from build123d import *

# Parameters (mm, degrees)
SKETCH_1_W           = 80
SKETCH_1_H           = 75
EXTRUDE_1_DEPTH      = 15
EXTRUDE_2_REACH      = 175.759
EXTRUDE_2_END_RADIUS = 39
SKETCH_2_W           = 45
SKETCH_2_H           = 30
SKETCH_3_R           = 19
EXTRUDE_3_DEPTH      = 62
SKETCH_4_R           = 17.5
CUT_EXTRUDE_1_DEPTH  = 62
SKETCH_6_R           = 5
EXTRUDE_4_DEPTH      = 30
FILLET_1_R           = 3
SKETCH_7_R           = 1.6
CUT_EXTRUDE_3_DEPTH  = 62
SKETCH_5_W           = 78.155385632
SKETCH_5_H           = 2
CUT_EXTRUDE_4_DEPTH  = 62
SKETCH_8_R           = 11
CUT_EXTRUDE_5_DEPTH  = 62
SKETCH_9_R           = 2.5
CUT_EXTRUDE_6_DEPTH  = 118.917343932
SKETCH_10_R          = 2
CUT_EXTRUDE_7_DEPTH  = 118.917343932
SKETCH_11_R          = 2
SKETCH_11_R_2        = 2.5
SKETCH_11_R_3        = 11
CUT_EXTRUDE_8_DEPTH  = 28
SKETCH_12_W          = 72
SKETCH_12_H          = 29.5
EXTRUDE_6_DEPTH      = 2
SKETCH_13_R          = 1.5
CUT_EXTRUDE_9_DEPTH  = 2
SKETCH_14_R          = 1.55
CUT_EXTRUDE_10_DEPTH = 250


with BuildPart() as part:
    # 草图1 → 凸台-拉伸1 (new, symmetric)
    with BuildSketch(Plane(origin=(0, 0, 0), x_dir=(1, 0, 0), z_dir=(0, 1, 0))):
        with BuildLine():
            Line((-40, -37.5), (-40, 37.5))
            ThreePointArc((-40, 37.5), (-68.287857357, 0), (-40, -37.5))
        make_face()
        Rectangle(SKETCH_1_W, SKETCH_1_H)
        with BuildLine():
            Line((40, -37.5), (40, 37.5))
            ThreePointArc((40, 37.5), (62.5, 0), (40, -37.5))
        make_face()
    extrude(amount=EXTRUDE_1_DEPTH, both=True)

    # 凸台-拉伸2: up to this cylinder (the profile starts outside it)
    extrude_2_end = Plane(origin=(-29.287857357, 0, 0), z_dir=(0, -1, 0)) * Cylinder(EXTRUDE_2_END_RADIUS, 430.518, mode=Mode.PRIVATE)
    # 草图2 → 凸台-拉伸2 (add, up to the surface)
    with BuildSketch(Plane(origin=(-106.5, 0, 0), x_dir=(0, 0, -1), z_dir=(1, 0, 0)), mode=Mode.PRIVATE) as extrude_2_sk1:
        Rectangle(SKETCH_2_W, SKETCH_2_H)
    extrude_2_tool1 = extrude(extrude_2_sk1.sketch, amount=EXTRUDE_2_REACH, mode=Mode.PRIVATE) - extrude_2_end
    add(extrude_2_tool1.solids().sort_by_distance((-106.5, 0, 0))[0])

    # 草图3 → 凸台-拉伸3 (add)
    with BuildSketch(Plane.ZY.offset(106.5)):
        Circle(SKETCH_3_R)
    extrude(amount=-EXTRUDE_3_DEPTH)

    # 草图4 → 切除-拉伸1 (cut)
    with BuildSketch(Plane.ZY.offset(106.5)):
        Circle(SKETCH_4_R)
    extrude(amount=-CUT_EXTRUDE_1_DEPTH, mode=Mode.SUBTRACT)

    # 草图6 → 凸台-拉伸4 (add)
    with BuildSketch(Plane(origin=(0, 15, 0), x_dir=(1, 0, 0), z_dir=(0, 1, 0))):
        with Locations((-96.5, 26.5)):
            Circle(SKETCH_6_R)
        with Locations((-76.5, 26.5)):
            Circle(SKETCH_6_R)
    extrude_4 = extrude(amount=-EXTRUDE_4_DEPTH)

    # 圆角1
    fillet_1_edges = [part.edges().sort_by_distance(p)[0] for p in [
        (-99.5, 0, -22.5),
        (-93.5, 0, -22.5),
        (-73.5, 0, -22.5),
        (-79.5, 0, -22.5),
    ]]
    fillet(fillet_1_edges, radius=FILLET_1_R)

    # 镜向3: 凸台-拉伸4 across plane
    add(extrude_4.mirror(Plane.XY))

    # 草图7 → 切除-拉伸3 (cut)
    with BuildSketch(Plane(origin=(0, 15, 0), x_dir=(1, 0, 0), z_dir=(0, 1, 0))):
        with Locations(Location((-96.5, 26.5, 0), (0, 0, 270))):
            Circle(SKETCH_7_R)
        with Locations(Location((-76.5, 26.5, 0), (0, 0, 270))):
            Circle(SKETCH_7_R)
        with Locations(Location((-76.5, -26.5, 0), (0, 0, 270))):
            Circle(SKETCH_7_R)
        with Locations(Location((-96.5, -26.5, 0), (0, 0, 270))):
            Circle(SKETCH_7_R)
    extrude(amount=-CUT_EXTRUDE_3_DEPTH, mode=Mode.SUBTRACT)

    # 草图5 → 切除-拉伸4 (cut)
    with BuildSketch(Plane.ZY.offset(106.5)):
        Rectangle(SKETCH_5_W, SKETCH_5_H)
    extrude(amount=-CUT_EXTRUDE_4_DEPTH, mode=Mode.SUBTRACT)

    # 草图8 → 切除-拉伸5 (cut)
    with BuildSketch(Plane.XZ.offset(15)):
        with Locations(Location((0, 0, 0), (0, 0, 270))):
            Circle(SKETCH_8_R)
    extrude(amount=-CUT_EXTRUDE_5_DEPTH, mode=Mode.SUBTRACT)

    # 草图9 → 切除-拉伸6 (cut, through all)
    with BuildSketch(Plane.XZ.offset(15)):
        with Locations(Location((14, 14, 0), (0, 0, 270))):
            Circle(SKETCH_9_R)
        with Locations(Location((14, -14, 0), (0, 0, 270))):
            Circle(SKETCH_9_R)
        with Locations(Location((-14, -14, 0), (0, 0, 270))):
            Circle(SKETCH_9_R)
        with Locations(Location((-14, 14, 0), (0, 0, 270))):
            Circle(SKETCH_9_R)
    extrude(amount=-CUT_EXTRUDE_6_DEPTH, mode=Mode.SUBTRACT)

    # 草图10 → 切除-拉伸7 (cut, through all)
    with BuildSketch(Plane(origin=(0, 15, 0), x_dir=(1, 0, 0), z_dir=(0, 1, 0))):
        with Locations(Location((32.5, 32.5, 0), (0, 0, 270))):
            Circle(SKETCH_10_R)
        with Locations(Location((-32.5, 32.5, 0), (0, 0, 270))):
            Circle(SKETCH_10_R)
        with Locations(Location((-32.5, -32.5, 0), (0, 0, 270))):
            Circle(SKETCH_10_R)
        with Locations(Location((32.5, -32.5, 0), (0, 0, 270))):
            Circle(SKETCH_10_R)
    extrude(amount=-CUT_EXTRUDE_7_DEPTH, mode=Mode.SUBTRACT)

    # 草图11 → 切除-拉伸8 (cut)
    with BuildSketch(Plane.XZ.offset(15)):
        with BuildLine():
            Line((-44.5, 9.013878189), (-44.5, 0))
            Line((-44.5, 0), (-44.5, -9.013878189))
            Line((-44.5, -9.013878189), (-44.5, -11.66190379))
            Line((-44.5, -11.66190379), (-44.5, -33.728188748))
            ThreePointArc((-44.5, -33.728188748), (-42.138664615, -34.696638927), (-39.716184164, -35.5))
            Line((-39.716184164, -35.5), (39.49358869, -35.5))
            ThreePointArc((39.49358869, -35.5), (60.5, 0), (39.49358869, 35.5))
            Line((39.49358869, 35.5), (-39.716184164, 35.5))
            ThreePointArc((-39.716184164, 35.5), (-42.138664615, 34.696638927), (-44.5, 33.728188748))
            Line((-44.5, 33.728188748), (-44.5, 11.66190379))
            Line((-44.5, 11.66190379), (-44.5, 9.013878189))
        make_face()
        with Locations(Location((-32.5, -32.5, 0), (0, 0, 90))):
            Circle(SKETCH_11_R, mode=Mode.SUBTRACT)
        with Locations(Location((-14, -14, 0), (0, 0, 270))):
            Circle(SKETCH_11_R_2, mode=Mode.SUBTRACT)
        with Locations(Location((32.5, -32.5, 0), (0, 0, 90))):
            Circle(SKETCH_11_R, mode=Mode.SUBTRACT)
        with Locations(Location((14, -14, 0), (0, 0, 270))):
            Circle(SKETCH_11_R_2, mode=Mode.SUBTRACT)
        with Locations(Location((0, 0, 0), (0, 0, 270))):
            Circle(SKETCH_11_R_3, mode=Mode.SUBTRACT)
        with Locations(Location((-14, 14, 0), (0, 0, 270))):
            Circle(SKETCH_11_R_2, mode=Mode.SUBTRACT)
        with Locations(Location((-32.5, 32.5, 0), (0, 0, 90))):
            Circle(SKETCH_11_R, mode=Mode.SUBTRACT)
        with Locations(Location((14, 14, 0), (0, 0, 270))):
            Circle(SKETCH_11_R_2, mode=Mode.SUBTRACT)
        with Locations(Location((32.5, 32.5, 0), (0, 0, 90))):
            Circle(SKETCH_11_R, mode=Mode.SUBTRACT)
    extrude(amount=-CUT_EXTRUDE_8_DEPTH, mode=Mode.SUBTRACT)

    # 草图12 → 凸台-拉伸6 (add)
    with BuildSketch(Plane.XZ.offset(15)):
        with BuildLine():
            Line((-44.5, 11.66190379), (-44.5, -11.66190379))
            Line((-44.5, -11.66190379), (-44.5, -33.728188748))
            ThreePointArc((-44.5, -33.728188748), (-42.138664615, -34.696638927), (-39.716184164, -35.5))
            Line((-39.716184164, -35.5), (39.49358869, -35.5))
            ThreePointArc((39.49358869, -35.5), (60.5, 0), (39.49358869, 35.5))
            Line((39.49358869, 35.5), (-39.716184164, 35.5))
            ThreePointArc((-39.716184164, 35.5), (-42.138664615, 34.696638927), (-44.5, 33.728188748))
            Line((-44.5, 33.728188748), (-44.5, 11.66190379))
        make_face()
        Rectangle(SKETCH_12_W, SKETCH_12_H, mode=Mode.SUBTRACT)
    extrude(amount=-EXTRUDE_6_DEPTH)

    # 草图13 → 切除-拉伸9 (cut)
    with BuildSketch(Plane.XZ.offset(15)):
        with Locations(Location((-44.75, 19, 0), (0, 0, 270))):
            Circle(SKETCH_13_R)
        with Locations(Location((0, 19, 0), (0, 0, 270))):
            Circle(SKETCH_13_R)
        with Locations(Location((44.75, 19, 0), (0, 0, 270))):
            Circle(SKETCH_13_R)
        with Locations(Location((44.75, -19, 0), (0, 0, 270))):
            Circle(SKETCH_13_R)
        with Locations(Location((0, -19, 0), (0, 0, 270))):
            Circle(SKETCH_13_R)
        with Locations(Location((-44.75, -19, 0), (0, 0, 270))):
            Circle(SKETCH_13_R)
    extrude(amount=-CUT_EXTRUDE_9_DEPTH, mode=Mode.SUBTRACT)

    # 草图14 → 切除-拉伸10 (cut, symmetric)
    with BuildSketch(Plane(origin=(0, 0, 0), x_dir=(1, 0, 0), z_dir=(0, 1, 0))):
        with Locations(Location((-66.5, 0, 0), (0, 0, 270))):
            Circle(SKETCH_14_R)
    extrude(amount=CUT_EXTRUDE_10_DEPTH, both=True, mode=Mode.SUBTRACT)


solid = part.part
Geometry check sheet. Reference: the model listing, model coordinates, mm. A direction names the side the tool comes from. Round coordinates to 2 decimals unless told otherwise and drop trailing zeros. Order: outer loops, then holes, each group sorted by start corner. A loop starts at its lowest first (then second) coordinate and runs counter-clockwise, first axis right, second up. Notation, with made-up numbers: (25.25, 59.5) -> (84.25, 59.5) arc R19 cw to (84.25, 87.5) -> close; hole circle Ø8 at (3.5, 25). An arc over 180 degrees is marked (long way). Use one line per item in the form item = value.
1. Go/stop test with flat-tipped pins: pin 1 (2.5 mm diameter, centred on x = 0, z = -19, fed in from -Y); pin 2 (10 mm diameter, centred on y = 5, z = -26.5, fed in from +X); pin 3 (3.5 mm diameter, centred on x = -96.5, z = -26.5, fed in from -Y). Record where each tip stops, or that it passes through.
Working result:
pin_1 = 13
pin_2 = 56.66
pin_3 = -15
2. Cross-section at B-B, the plane x = 49. Enter the section's corners in (y, z).
Working result:
outline = (-15, -31.07) -> (15, -31.07) -> (15, 31.07) -> (-15, 31.07) -> close; hole (-13, -28.27) -> (13, -28.27) -> (13, 28.27) -> (-13, 28.27) -> close
3. Mould release check, pull along Y, two halves, no side actions. Record for faces 1 (the face through (-102.2, 8.1, -23.5)), 2 (the face through (-76, 1, 22)), 3 (the face through (-23, 15, 1)): pulls with the +Y half, pulls with the -Y half, needs draft (parallel to the pull), parting line crosses it, or undercut.
Working result:
face_1 = needs draft
face_2 = undercut
face_3 = pulls with the +Y half
4. Cross-section at D-D, the plane x = -66.5. Enter the section's corners in (y, z).
Working result:
outline = (-18.94, -1.55) arc R19 ccw to (-15, -11.66) -> (-15, -22.5) -> (-1, -22.5) -> (-1, -17.47) arc R17.5 cw to (-17.43, -1.55) -> close; (-18.94, 1.55) -> (-17.43, 1.55) arc R17.5 cw to (-1, 17.47) -> (-1, 22.5) -> (-15, 22.5) -> (-15, 11.66) arc R19 ccw to start; (1, -22.5) -> (15, -22.5) -> (15, -11.66) arc R19 ccw to (18.94, -1.55) -> (17.43, -1.55) arc R17.5 cw to (1, -17.47) -> close; (1, 17.47) arc R17.5 cw to (17.43, 1.55) -> (18.94, 1.55) arc R19 ccw to (15, 11.66) -> (15, 22.5) -> (1, 22.5) -> close
5. Set-up check for faces 4 (the face through (-82.2, -7.9, -23.5)), 5 (the face through (30.726, 14.014, 33.423)), 6 (the face through (-42.172, -0.182, -34.684)): record each of +Z, -Z, +X, -X, +Y, -Y from which the full face is reachable in a straight line by a thin tool's end or side.
Working result:
face_4 = +Y, -Y
face_5 = +Y
face_6 = none
6. Scan lines: line 1 along Z through (x, y) = (-32.5, 13.8); line 2 along Y through (x, z) = (-74.5, 1); line 3 along Z through (x, y) = (-29, -11.5). Record each from-to range of solid material in increasing order. Write a range as from..to.
Working result:
line_1 = -37.5..-34.5, -30.5..30.5, 34.5..37.5
line_2 = -18.97..-17.47, 17.47..18.97
line_3 = -37.5..-35.5, 35.5..37.5
7. Cross-section at C-C, the plane y = 4. Count the separate pieces of the cut face and the enclosed holes in it, plus the area to 3 significant figures.
Working result:
separate_pieces = 1
enclosed_holes = 4
area = 1,740 mm^2
8. Cross-section at A-A, the plane x = -32.5. Enter the section's corners in (y, z), plus the area to 3 significant figures.
Working result:
outline = (-15, -37.5) -> (15, -37.5) -> (15, -34.5) -> (13, -34.5) -> (13, -35.5) -> (-13, -35.5) -> (-13, -14.75) -> (-15, -14.75) -> close; (-15, 14.75) -> (-13, 14.75) -> (-13, 35.5) -> (13, 35.5) -> (13, 34.5) -> (15, 34.5) -> (15, 37.5) -> (-15, 37.5) -> close; (13, -30.5) -> (15, -30.5) -> (15, 30.5) -> (13, 30.5) -> close
area = 329 mm^2
